from build123d import *

# Parameters (mm, degrees)
SKETCH1_W            = 93.98
SKETCH1_H            = 50.8
BOSS_EXTRUDE4_DEPTH  = 3.81
SKETCH26_W           = 3.048
SKETCH26_H           = 3.048
CUT_EXTRUDE30_DEPTH  = 54.551248351
LPATTERN9_COUNT      = 4
LPATTERN9_PITCH      = 12.7
LPATTERN9_COUNT_DIR2 = 7
LPATTERN9_PITCH_DIR2 = 12.7
SKETCH25_R           = 1.524
SKETCH25_R_2         = 0.8
CUT_EXTRUDE29_DEPTH  = 54.551248351
SKETCH27_W           = 15.24
SKETCH27_H           = 3.81
BOSS_EXTRUDE5_DEPTH  = 3.81
SKETCH28_R           = 1.524
CUT_EXTRUDE31_DEPTH  = 56.459898125


with BuildPart() as part:
    # Sketch1 → Boss-Extrude4 (new body)
    with BuildSketch(Plane.XY):
        Rectangle(SKETCH1_W, SKETCH1_H)
    extrude(amount=BOSS_EXTRUDE4_DEPTH)

    # Sketch26 → Cut-Extrude30 (cut, through all)
    with BuildSketch(Plane.XY.offset(3.81)):
        with Locations((38.1, 19.05)):
            Rectangle(SKETCH26_W, SKETCH26_H)
    cut_extrude30 = extrude(amount=-CUT_EXTRUDE30_DEPTH, mode=Mode.SUBTRACT)

    # LPattern9: Cut-Extrude30 4 × 7
    with Locations(*[(-j * LPATTERN9_PITCH_DIR2, -i * LPATTERN9_PITCH, 0) for i in range(LPATTERN9_COUNT) for j in range(LPATTERN9_COUNT_DIR2) if (i, j) != (0, 0)]):
        add(cut_extrude30, mode=Mode.SUBTRACT)

    # Sketch25 → Cut-Extrude29 (cut, through all)
    with BuildSketch(Plane.XY.offset(3.81)):
        with Locations((0, -12.7)):
            Circle(SKETCH25_R)
        with Locations((-4.572, -12.7)):
            Circle(SKETCH25_R_2)
        with Locations((4.572, -12.7)):
            Circle(SKETCH25_R_2)
    extrude(amount=-CUT_EXTRUDE29_DEPTH, mode=Mode.SUBTRACT)

    # Sketch27 → Boss-Extrude5 (add)
    with BuildSketch(Plane.XY.offset(3.81)):
        with Locations((25.4, 27.305)):
            Rectangle(SKETCH27_W, SKETCH27_H)
    boss_extrude5 = extrude(amount=-BOSS_EXTRUDE5_DEPTH)

    # Sketch28 → Cut-Extrude31 (cut, through all)
    with BuildSketch(Plane.XY.offset(3.81)):
        with Locations((25.4, 26.924)):
            Circle(SKETCH28_R)
    cut_extrude31 = extrude(amount=-CUT_EXTRUDE31_DEPTH, mode=Mode.SUBTRACT)

    # Mirror1: Boss-Extrude5, Cut-Extrude31 across plane
    add(boss_extrude5.mirror(Plane(origin=(0, 0, 0), x_dir=(0, 0, 1), z_dir=(1, 0, 0))))
    add(cut_extrude31.mirror(Plane(origin=(0, 0, 0), x_dir=(0, 0, 1), z_dir=(1, 0, 0))), mode=Mode.SUBTRACT)


solid = part.part
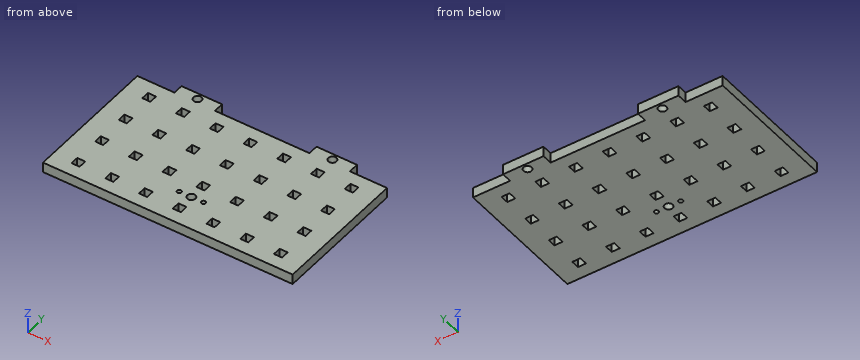
Part model, mm, in its own coordinate system. Coordinates: 2 decimals unless noted, no trailing zeros. Loops run counter-clockwise (first coordinate to the right, second up) from the corner with the lowest first, then second, coordinate; pieces in that order, holes last. Notation, with made-up numbers: M 87,7.5 L 111,7.5 A32 ccw 111,43.5 Z; hole C 21.5,21.25 d10. An arc over 180 degrees is marked long. Use a Markdown table: item, result. Add a question column.
Q1. Cut at C-C (x = 25.4). Write the cut outline in (y, z), and give its area (3 significant figures).
Q2. Cut at A-A (x = 0). Write the cut outline in (y, z).
Q3. Pin check, flat tips, straight feed: P1, Ø0.9, axis at x = -12.5, z = 1, coming from the +Y side; P2, Ø4, axis at x = 33, y = 9.5, coming from the -Z side. Stop position of each tip, or through.
Q4. Probe L1, parallel to Y at x = 37, z = 2.8; L2, parallel to Y at x = 0, z = 1.9; L3, parallel to X at y = -12, z = 2.85. List the from-to ranges inside material, lowest first.
Q5. Cut at B-B (z = 0.85). Give the number of separate pieces and of enclosed holes in the cut face, and give its area (3 significant figures).
Worked out:
| question | item | result |
|---|---|---|
| 1 | outline | M -25.4,0 L -20.57,0 L -20.57,3.81 L -25.4,3.81 Z; M -17.53,0 L -7.87,0 L -7.87,3.81 L -17.53,3.81 Z; M -4.83,0 L 4.83,0 L 4.83,3.81 L -4.83,3.81 Z; M 7.87,0 L 17.53,0 L 17.53,3.81 L 7.87,3.81 Z; M 20.57,0 L 25.4,0 L 25.4,3.81 L 20.57,3.81 Z; M 28.45,0 L 29.21,0 L 29.21,3.81 L 28.45,3.81 Z |
| 1 | area | 150 mm2 |
| 2 | outline | M -25.4,0 L -20.57,0 L -20.57,3.81 L -25.4,3.81 Z; M -17.53,0 L -14.22,0 L -14.22,3.81 L -17.53,3.81 Z; M -11.18,0 L -7.87,0 L -7.87,3.81 L -11.18,3.81 Z; M -4.83,0 L 4.83,0 L 4.83,3.81 L -4.83,3.81 Z; M 7.87,0 L 17.53,0 L 17.53,3.81 L 7.87,3.81 Z; M 20.57,0 L 25.4,0 L 25.4,3.81 L 20.57,3.81 Z |
| 3 | P1 | stops at y = 25.4 |
| 3 | P2 | stops at z = 0 |
| 4 | L1 | y = -25.4 to -20.57, -17.53 to -7.87, -4.83 to 4.83, 7.87 to 17.53, 20.57 to 25.4 |
| 4 | L2 | y = -25.4 to -20.57, -17.53 to -14.22, -11.18 to -7.87, -4.83 to 4.83, 7.87 to 17.53, 20.57 to 25.4 |
| 4 | L3 | x = -46.99 to -4.96, -4.18 to -1.35, 1.35 to 4.18, 4.96 to 46.99 |
| 5 | separate pieces | 1 |
| 5 | enclosed holes | 33 |
| 5 | area | 4,600 mm2 |
